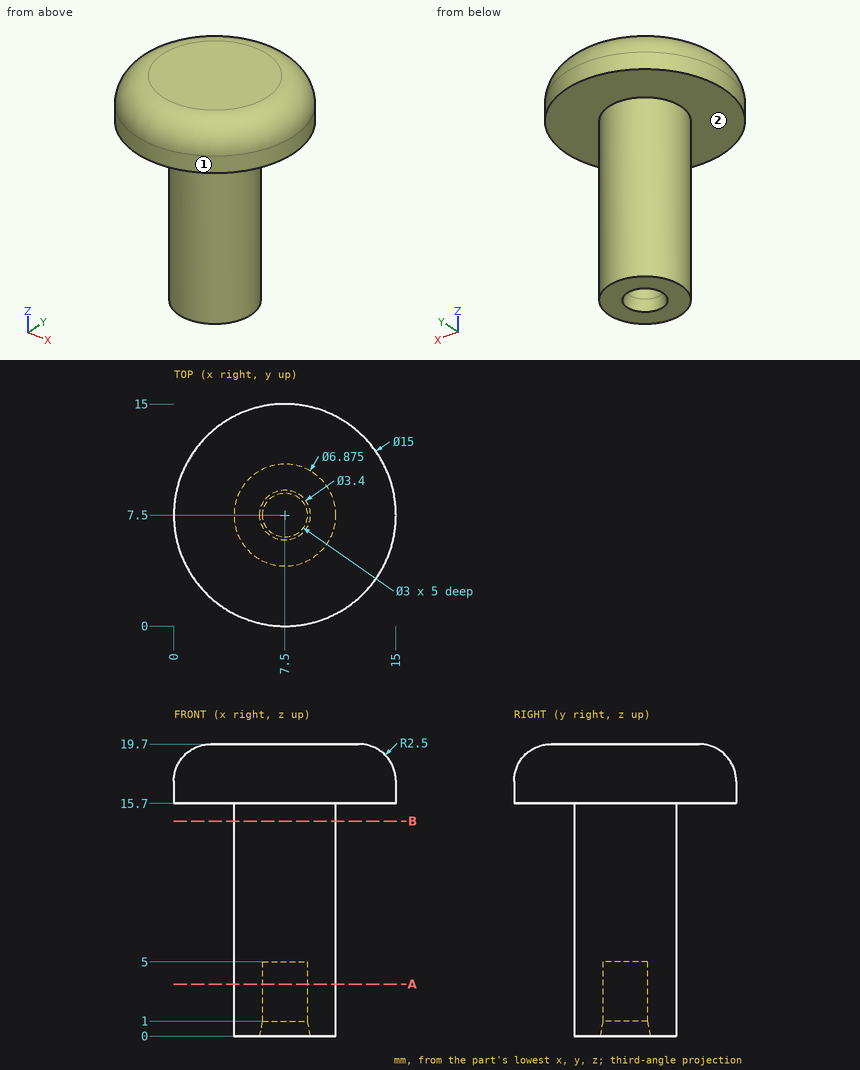
Print and shaded views of the part. All mm, measured from the part's lowest x, y and z. A direction names the side the tool comes from. Coordinates: 2 decimals unless noted, no trailing zeros. Order: outer loops, then holes, each group sorted by start corner. A loop starts at its lowest first (then second) coordinate and runs counter-clockwise, first axis right, second up. Notation, with made-up numbers: M 43,-39 L 66,-39 A22 cw 66,-21 Z; hole C 3.5,-31.75 d5. An arc over 180 degrees is marked long. Answer as CSV lines item,"result".
1) Drill centre lines: L1, parallel to Y at x = 7.5, z = 1.95; L2, parallel to Z at x = 12.25, y = 9.5; L3, parallel to Z at x = 6.75, y = 6.5. Where is each one in solid material? Low to high. Write a range as from..to.
Verdict:
L1,"4.06..6, 9..10.94"
L2,"15.7..19.7"
L3,"5..19.7"
2) 3-axis set-ups, long thin cutter, end or side, ignore diameter. For the marked faces 1 and 2: which of +Z, -Z, +X, -X, +Y, -Y reach the whole face in a straight line?
Verdict:
face 1,"+Z, -Z"
face 2,"-Z"
3) Flat gauge pins, fed straight in: P1, Ø3, axis at y = 9.5, z = 15.5, coming from the -X side; P2, Ø1.8, axis at x = 7.5, y = 7.5, coming from the -Z side; P3, Ø5, axis at x = 7, z = 7, coming from the +Y side. Where does each tip first touch, or does it go through?
Verdict:
P1,"x = 0.02"
P2,"z = 5"
P3,"y = 10.94"
4) Cut at A-A (z = 3.5). List the corners of the cut face in (x, y) (1 decimal).
Verdict:
outline,"C 7.5,7.5 d6.9; hole C 7.5,7.5 d3"
5) Cut at B-B (z = 14.5). List the corners of the cut face in (x, y) (1 decimal).
Verdict:
outline,"C 7.5,7.5 d6.9"
